from build123d import *

# Parameters (mm, degrees)
SKETCH_7_R          = 1.6
SKETCH_7_W          = 15
SKETCH_7_H          = 10
EXTRUDE_1_DEPTH     = 4
SKETCH_8_R          = 1.6
CUT_EXTRUDE_1_DEPTH = 4
SKETCH_7_3_W        = 15
SKETCH_7_3_H        = 10
EXTRUDE_2_DEPTH     = 5
CUT_EXTRUDE_2_DEPTH = 5


with BuildPart() as part:
    # 草图7 → 凸台-拉伸1 (new body)
    # profile 1 of 3: a face of its own
    with BuildSketch(Plane(origin=(0, 0, 0), x_dir=(1, 0, 0), z_dir=(0, 1, 0))):
        Polygon((33, 23.6), (-33, 23.6), (-33, 14.5), (-18, 14.5), (-18, 4.5), (-33, 4.5), (-33, -23.6), (33, -23.6), (33, -14.5), (18, -14.5), (18, -4.5), (33, -4.5), align=None)
        with Locations(Location((-27.5, -17.5, 0), (0, 0, 270))):
            Circle(SKETCH_7_R, mode=Mode.SUBTRACT)
        with Locations(Location((27.5, -17.5, 0), (0, 0, 270))):
            Circle(SKETCH_7_R, mode=Mode.SUBTRACT)
        with Locations(Location((-27.5, 17.5, 0), (0, 0, 270))):
            Circle(SKETCH_7_R, mode=Mode.SUBTRACT)
        with Locations(Location((27.5, 17.5, 0), (0, 0, 270))):
            Circle(SKETCH_7_R, mode=Mode.SUBTRACT)
    # profile 2 of 3: a face of its own
    with BuildSketch(Plane(origin=(0, 0, 0), x_dir=(1, 0, 0), z_dir=(0, 1, 0))):
        with Locations((-25.5, 9.5)):
            Rectangle(SKETCH_7_W, SKETCH_7_H)
    # profile 3 of 3: a face of its own
    with BuildSketch(Plane(origin=(0, 0, 0), x_dir=(1, 0, 0), z_dir=(0, 1, 0))):
        with Locations((25.5, -9.5)):
            Rectangle(SKETCH_7_W, SKETCH_7_H)
    extrude(amount=EXTRUDE_1_DEPTH)

    # 草图8 → 切除-拉伸1 (cut)
    with BuildSketch(Plane.XZ):
        with Locations(Location((-5.25, -16.6, 0), (0, 0, 270))):
            Circle(SKETCH_8_R)
        with Locations(Location((5.25, -16.6, 0), (0, 0, 270))):
            Circle(SKETCH_8_R)
        with Locations(Location((-5.25, 16.6, 0), (0, 0, 90))):
            Circle(SKETCH_8_R)
        with Locations(Location((5.25, 16.6, 0), (0, 0, 90))):
            Circle(SKETCH_8_R)
    extrude(amount=-CUT_EXTRUDE_1_DEPTH, mode=Mode.SUBTRACT)

    # 草图7<3> → 凸台-拉伸2 (add)
    with BuildSketch(Plane(origin=(0, 0, 0), x_dir=(1, 0, 0), z_dir=(0, 1, 0))):
        with Locations((-25.5, 9.5)):
            Rectangle(SKETCH_7_3_W, SKETCH_7_3_H)
        with Locations((25.5, -9.5)):
            Rectangle(SKETCH_7_3_W, SKETCH_7_3_H)
    extrude(amount=-EXTRUDE_2_DEPTH)

    # 草图10 → 切除-拉伸2 (cut)
    with BuildSketch(Plane.XZ):
        with BuildLine():
            ThreePointArc((-23.130789545, -14.5), (-27.5, -12.2), (-31.869210455, -14.5))
            Line((-31.869210455, -14.5), (-23.130789545, -14.5))
        make_face()
        with BuildLine():
            ThreePointArc((23.130789545, 14.5), (27.5, 12.2), (31.869210455, 14.5))
            Line((31.869210455, 14.5), (23.130789545, 14.5))
        make_face()
    extrude(amount=CUT_EXTRUDE_2_DEPTH, mode=Mode.SUBTRACT)


solid = part.part
Geometry check sheet. Reference: the model listing, model coordinates, mm. A direction names the side the tool comes from. Round coordinates to 2 decimals unless told otherwise and drop trailing zeros. Write each loop counter-clockwise with the first axis right and the second up, starting at its lowest first coordinate (ties: lowest second). Pieces come first, ordered by that corner, then holes. Notation, with made-up numbers: (52, 6.5) -> (60, 6.5) arc R18 ccw to (60, 19.5) -> close; hole circle Ø7 at (84.25, -2). An arc over 180 degrees is marked (long way). One line per item, written item: value. Start each with the question number.
(1) Cross-section at A-A, the plane x = 5.25. Record the cut outline in (y, z).
(2) Access from +Z, -Z, +X, -X, +Y, -Y to the whole of each face (thin tool, end or side, straight path). Record for faces 4 (the cylindrical face through (-27.4, -2.5, -12.2)), 5 (the flat face through (18, -2, 10)), 6 (the flat face through (-26, -2, -4.5)), 7 (the flat face through (25, -2, 4.5)), 8 (the cylindrical face through (27.4, -2.5, 12.2)).
(3) Go/stop test with flat-tipped pins: pin 1 Ø1.5 at (x, z) = (12, -8.5) entering from -Y; pin 2 Ø2.5 at (x, y) = (-26.5, -3) entering from +Z; pin 3 Ø1.5 at (y, z) = (-2, 7.5) entering from -X; pin 4 Ø3 at (x, y) = (-14, -1) entering from -Z. Record where each tip stops, or that it passes through.
(4) Draft check along Z on faces 1 (the flat face through (-26, -5, -10)), 2 (the cylindrical face through (4.64, 1.97, -18.08)), 3 (the flat face through (0, 2, -23.6)). Enter one of: +Z half, -Z half, draft (parallel to the pull), parting line (faces both ways), or undercut.
(5) Cross-section at C-C, the plane z = 16.6. Record the cut outline in (x, y), and give its area (3 significant figures).
(6) Cross-section at B-B, the plane y = -2.25. Record the cut outline in (x, z).
(7) Scan lines: line 1 (X direction, y = 2.45, z = 17.5); line 2 (Y direction, x = 11, z = 10); line 3 (X direction, y = 1.05, z = 16.6). Record each from-to range of solid material in increasing order. Write a range as [from, to].
(8) Cross-section at D-D, the plane x = 27.5. Record the cut outline in (y, z), and give its area (3 significant figures).
Answer:
1. outline: (0, -23.6) -> (4, -23.6) -> (4, -18.2) -> (0, -18.2) -> close; (0, -15) -> (4, -15) -> (4, 15) -> (0, 15) -> close; (0, 18.2) -> (4, 18.2) -> (4, 23.6) -> (0, 23.6) -> close
2. face 4: -Z, -Y
2. face 5: +Z, -Z, -X, -Y
2. face 6: +Z, +X, -X, -Y
2. face 7: -Z, +X, -X, -Y
2. face 8: +Z, -Y
3. pin 1: y = 0
3. pin 2: z = -4.5
3. pin 3: x = 18
3. pin 4: z = -23.6
4. face 1: draft
4. face 2: undercut
4. face 3: -Z half
5. outline: (-33, 0) -> (-28.82, 0) -> (-28.82, 4) -> (-33, 4) -> close; (-26.18, 0) -> (-6.85, 0) -> (-6.85, 4) -> (-26.18, 4) -> close; (-3.65, 0) -> (3.65, 0) -> (3.65, 4) -> (-3.65, 4) -> close; (6.85, 0) -> (26.18, 0) -> (26.18, 4) -> (6.85, 4) -> close; (28.82, 0) -> (33, 0) -> (33, 4) -> (28.82, 4) -> close
5. area: 217 mm²
6. outline: (-33, -14.5) -> (-31.87, -14.5) arc R5.3 cw to (-23.13, -14.5) -> (-18, -14.5) -> (-18, -4.5) -> (-33, -4.5) -> close; (18, 4.5) -> (33, 4.5) -> (33, 14.5) -> (31.87, 14.5) arc R5.3 cw to (23.13, 14.5) -> (18, 14.5) -> close
7. line 1: [-33, -29.1], [-25.9, -6.57], [-3.93, 3.93], [6.57, 25.9], [29.1, 33]
7. line 2: [0, 4]
7. line 3: [-33, -28.82], [-26.18, -6.85], [-3.65, 3.65], [6.85, 26.18], [28.82, 33]
8. outline: (-5, 4.5) -> (0, 4.5) -> (0, -15.9) -> (4, -15.9) -> (4, 15.9) -> (0, 15.9) -> (0, 12.2) -> (-5, 12.2) -> close; (0, -23.6) -> (4, -23.6) -> (4, -19.1) -> (0, -19.1) -> close; (0, 19.1) -> (4, 19.1) -> (4, 23.6) -> (0, 23.6) -> close
8. area: 202 mm²
